Source: CAD feature listing. Evaluate the final solid. Frame: model axes, mm. Face numbers are marked on the shaded views. A direction names the side the tool comes from. Give positions to 0.01 mm unless a question says otherwise; leave off trailing zeros. Loops run counter-clockwise (first coordinate to the right, second up) from the corner with the lowest first, then second, coordinate; pieces in that order, holes last.
Autodesk Inventor part; units mm, degrees
ref_plane "Work Plane1" through (30, 0, 0) normal (0, -0.5, 0.8660254) x (1, 0, 0)
ref_plane "YZ Plane" through (0, 0, 0) normal (1, 0, 0) x (0, 1, 0)
ref_plane "XZ Plane" through (0, 0, 0) normal (0, 1, 0) x (-1, 0, 0)
sketch "Эскиз1" plane through (0, 0, 0) normal (0, 0, 1) x (1, 0, 0)
  line L0 (-0.0667, 0) -> (20, 0)
  line L1 (20, 0) -> (20, 2)
  line L2 (20, 2) -> (1.4, 2)
  line L3 (1.4, 2) -> (0.9706, 2)
  line L4 (0.9706, 2) -> (0, 2)
  line L5 (0, 2) -> (0, 3.8)
  line L6 (0, 3.8) -> (-2.2, 3.8)
  line L7 (-2.2, 3.8) -> (-2.2, 1.4434)
  line L8 (-2.2, 1.4434) -> (-0.9, 1.4434)
  line L9 (-0.9, 1.4434) -> (-0.0667, 0)
  line L10 (-6.64, 0) -> (24.44, 0)
  line L11 (0, -0.76) -> (0, 4.56)
  line L12 (1.4, 2) -> (0, 2) construction
  dimension "d0" = 18.6
  dimension "d1" = 0.4294
  dimension "d2" = 2.2
  dimension "d3" = 1.3
  dimension "d4" = 60
  dimension "d5" = 4
  dimension "d6" = 4
  dimension "d7" = 2.8868
  dimension "d8" = 7.6
  dimension "d19" = 20
revolve "Базовый элемент" add sketch "Эскиз1" angle 360 about axis through (-0.0667, 0, 0) along (1, 0, 0)
sketch "Эскиз2" plane through (-2.2, 0, 0) normal (-1, 0, 0) x (0, 0, 1)
  circle A0 centre (0, 0) radius 1.4434
  line L0 (0, -5.32) -> (0, 5.32)
  line L1 (-5.32, 0) -> (5.32, 0)
  line L2 (1.4434, 0) -> (0.7217, -1.25)
  line L3 (0.7217, -1.25) -> (-0.7217, -1.25)
  line L4 (-0.7217, -1.25) -> (-1.4434, 0)
  line L5 (-1.4434, 0) -> (-0.7217, 1.25)
  line L6 (-0.7217, 1.25) -> (0.7217, 1.25)
  line L7 (0.7217, 1.25) -> (1.4434, 0)
  point P0 (0, 0)
extrude "Паз" add sketch "Эскиз2" against normal up to next contours L7 A0 | A0 L2 | L6 L0 A0 | A0 L0 L3 | L0 L6 A0 | A0 L3 L0 | L4 A0 | A0 L5
fillet "Сопряжение1" radius 1.9 1 edges at (-2.2, -3.8, 0)
thread "Резьба"
chamfer "Фаска1" distance 0.4294 distance2 0.4294 1 edges at (20, -2, 0) measured on face at (20, 0.527, -0.2661)
fillet "Сопряжение2" radius 0.2 1 edges at (0, -2, 0)
ref_plane "Work Plane1" through (30, 0, 0) normal (0, -0.5, 0.8660254) x (1, 0, 0)
equation "\"d0\" = GEL"
equation "\"d1\" = GAL"
equation "\"d2\" = KOH"
equation "\"d3\" = INTI"
equation "\"d5\" = GD"
equation "\"d6\" = BDM"
equation "\"d7\" = 1.1547 * SW"
equation "\"d8\" = KOD"
equation "\"d19\" = NLG"
equation "\"d16\" = RR"
equation "\"d12\" = GEL"
equation "\"d14\" = -0.5 * SPD + 0.5 * GD"
equation "\"d15\" = GUL"
equation "\"d29\" = R"
equation "\"GD\" = NND"
equation "\"NLG\" = 20"
equation "\"GEL\" = 18.6"
equation "\"KOD\" = 7.6"
equation "\"KOH\" = 2.2"
equation "\"INTI\" = 1.3"
equation "\"GAL\" = 0.61345 * PTC"
equation "\"GUL\" = 0.61345 * PTC"
equation "\"BDM\" = NND"
equation "\"SW\" = 2.5"
equation "\"RR\" = 1.9"
equation "\"SPD\" = 3.14117"
equation "\"d28\" = R"
equation "\"R\" = 0.2"
equation "\"TOA\" = 30deg"
equation "\"THREADDIA\" = 4"
equation "\"KOD1\" = KOD - 2 * RR"
equation "\"PTC\" = 0.7"
equation "\"NND\" = 4"
equation "\"E0\" = 1.155 * SW"
equation "\"GD1\" = THREADDIA - 1.2269 * PTC"
properties part number "ANSI B18.3.4M - M4 x 0.7 x 20, BHSBHCSM" material "Сталь, мягкая"
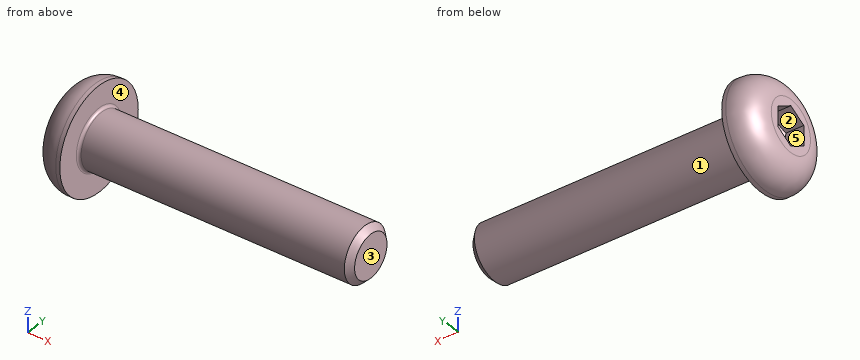
1) Pull-direction query (Z, two-part tool) for the marked faces 1, 2 and 3; classes: released by +Z, released by -Z, zero draft, split by the parting line, or undercut.
Checks:
face 1: split by the parting line
face 2: undercut
face 3: zero draft
2) Reachability of the marked faces 4 and 5 from +Z, -Z, +X, -X, +Y, -Y: full face, straight path, thin tool, end or side. Return the list, or none.
Checks:
face 4: +X
face 5: -X
3) Contact query for flat-ended pins moving along their axis: P1, Ø4, axis at x = 6.5, z = -1.5, coming from the -Y side; P2, Ø3, axis at y = 2.5, z = 2, coming from the +X side; P3, Ø1, axis at x = 6, z = 3, coming from the -Y side; P4, Ø4, axis at y = -3, z = 3, coming from the +X side. Output: stop coordinate, or through.
Checks:
P1: stops at y = -2
P2: stops at x = 19.87
P3: passes through
P4: stops at x = 0
4) Cut plane A-A (x = 14.75). Return loops of the section in (y, z), and give its area (3 significant figures).
Checks:
outline: circle Ø4 at (0, 0)
area: 12.6 mm2
5) Ray query, probe 1 along X at (y, z) = (-2.5, -1); probe 2 along Y at (x, z) = (10, -1); probe 3 along Y at (x, z) = (17.75, -1.75). Return the intervals inside material, ascending.
Checks:
probe 1: x = -2.03 to 0
probe 2: y = -1.73 to 1.73
probe 3: y = -0.97 to 0.97
